Here's how the part is built. I have some questions about the finished solid (model axes, mm). Coordinates: 2 decimals unless noted, no trailing zeros. Write each loop counter-clockwise with the first axis right and the second up, starting at its lowest first coordinate (ties: lowest second). Pieces come first, ordered by that corner, then holes. Notation, with made-up numbers: (51.25, 10) -> (68.25, 10) arc R11 ccw to (68.25, 18) -> close; hole circle Ø1 at (75, 72.25). An arc over 180 degrees is marked (long way). Put each result on its own line as item: value. Start each with the question number.
Item 1: If we mould it in two halves opening along X, with no side actions, what happens to faces 1 (the face through (0, 3, 3)), 2 (the face through (14.63, 2.51, -0.04)), 3 (the face through (17.5, 3, 0))? For each: released by +X, released by -X, zero draft, split by the parting line, or undercut.
Item 2: I need wall thicknesses on line 1 (Z direction, x = -9.5, y = 3.1); line 2 (Y direction, x = -6, z = 1.2); line 3 (Z direction, x = 9, y = 3.4). Which ranges of each line are inside material? Lowest first, please. Write a range as [from, to].
Item 3: I want a section at A-A, the plane y = 3. List the corners of the cut face in (x, z) for me, then the cut area to 3 significant figures.
Item 4: I want a section at C-C, the plane z = 0.5. List the corners of the cut face in (x, y) for me.
Item 5: I want a section at D-D, the plane y = 4.9. List the corners of the cut face in (x, z) for me, then the cut area to 3 significant figures.
Item 6: I want a section at B-B, the plane x = 14. List the corners of the cut face in (y, z) for me.
from build123d import *

# Parameters (mm, degrees)
SKETCH1_W             = 35
SKETCH1_H             = 6
BOSS_EXTRUDE1_DEPTH   = 5.5
M2X0_4_TAPPED_HOLE1_D = 1.6
M2X0_4_TAPPED_HOLE2_D = 1.6


with BuildPart() as part:
    # Sketch1 → Boss-Extrude1 (new body)
    with BuildSketch(Plane(origin=(0, 0, 0), x_dir=(1, 0, 0), z_dir=(0, 1, 0))):
        Rectangle(SKETCH1_W, SKETCH1_H)
    extrude(amount=BOSS_EXTRUDE1_DEPTH)

    # M2x0.4 Tapped Hole1 (through all)
    with Locations(Plane.XY.offset(3)):
        with Locations((6, 3), (-14, 3), (-6, 3), (14, 3)):
            Hole(M2X0_4_TAPPED_HOLE1_D / 2)

    # M2x0.4 Tapped Hole2 (through all)
    with Locations(Plane(origin=(0, 5.5, 0), x_dir=(-1, 0, 0), z_dir=(0, 1, 0))):
        with Locations((9.5, 0), (-9.5, 0)):
            Hole(M2X0_4_TAPPED_HOLE2_D / 2)


solid = part.part
Calculated:
1. face 1: zero draft
1. face 2: undercut
1. face 3: released by +X
2. line 1: z = [-3, -0.8], [0.8, 3]
2. line 2: y = [0, 2.2], [3.8, 5.5]
2. line 3: z = [-3, -0.62], [0.62, 3]
3. outline: (-17.5, -3) -> (-14.8, -3) -> (-14.8, 3) -> (-17.5, 3) -> close; (-13.2, -3) -> (-6.8, -3) -> (-6.8, 3) -> (-13.2, 3) -> close; (-5.2, -3) -> (5.2, -3) -> (5.2, 3) -> (-5.2, 3) -> close; (6.8, -3) -> (13.2, -3) -> (13.2, 3) -> (6.8, 3) -> close; (14.8, -3) -> (17.5, -3) -> (17.5, 3) -> (14.8, 3) -> close; hole circle Ø1.6 at (-9.5, 0); hole circle Ø1.6 at (9.5, 0)
3. area: 168 mm2
4. outline: (-17.5, 0) -> (-10.12, 0) -> (-10.12, 5.5) -> (-17.5, 5.5) -> close; (-8.88, 0) -> (8.88, 0) -> (8.88, 5.5) -> (-8.88, 5.5) -> close; (10.12, 0) -> (17.5, 0) -> (17.5, 5.5) -> (10.12, 5.5) -> close; hole circle Ø1.6 at (-14, 3); hole circle Ø1.6 at (-6, 3); hole circle Ø1.6 at (6, 3); hole circle Ø1.6 at (14, 3)
5. outline: (-17.5, -3) -> (17.5, -3) -> (17.5, 3) -> (-17.5, 3) -> close; hole circle Ø1.6 at (-9.5, 0); hole circle Ø1.6 at (9.5, 0)
5. area: 206 mm2
6. outline: (0, -3) -> (2.2, -3) -> (2.2, 3) -> (0, 3) -> close; (3.8, -3) -> (5.5, -3) -> (5.5, 3) -> (3.8, 3) -> close
